Study the drawing (mm; zero at the part's minimum x, y, z) and answer. A direction names the side the tool comes from. Coordinates: 2 decimals unless noted, no trailing zeros. Write each loop counter-clockwise with the first axis right and the second up, starting at its lowest first coordinate (ties: lowest second). Pieces come first, ordered by that corner, then holes. Notation, with made-up numbers: M 84.25,59 L 101.25,59 A23 cw 101.25,98 Z; hole C 72.25,21.25 d6. An arc over 180 degrees is marked long. Answer as a JSON object with one key per item and string values. Group by question number.
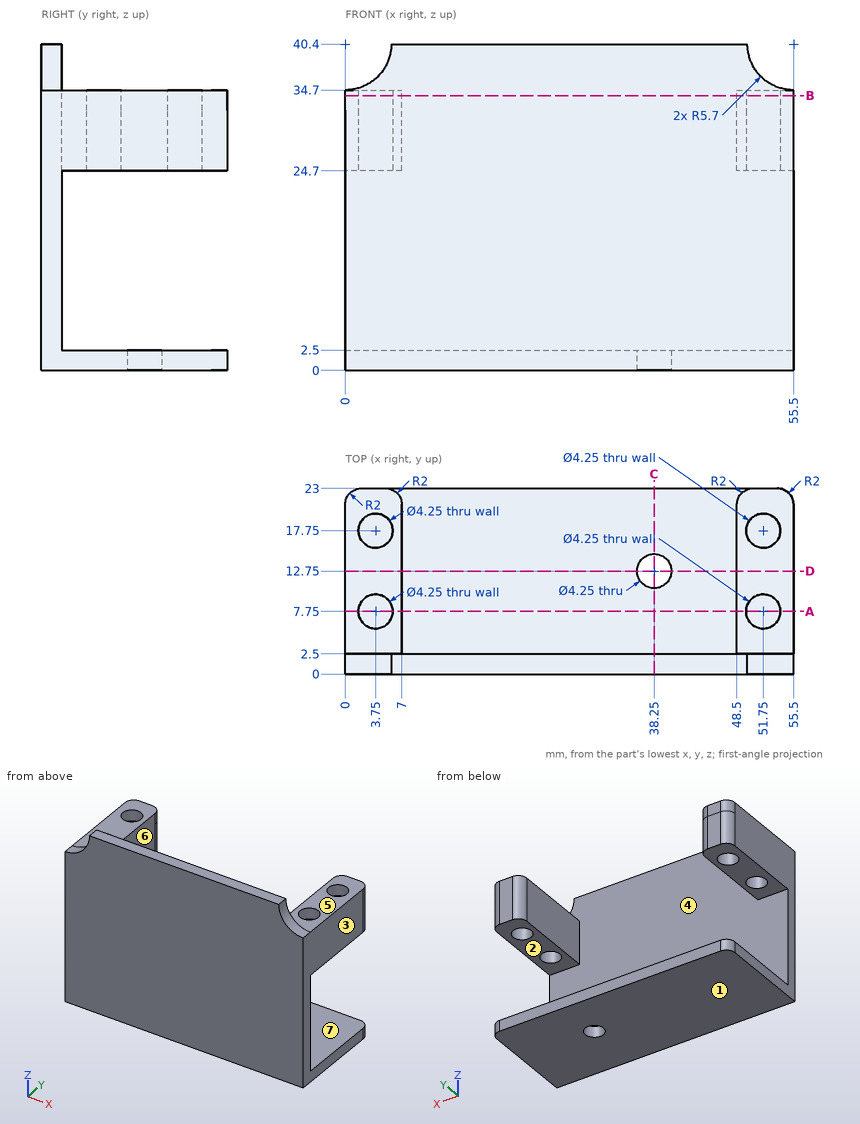
Item 1: Consider L1, parallel to X at y = 7.75, z = 26.5 (3 decimals); L2, parallel to Y at x = 3.75, z = 26.5 (3 decimals); L3, parallel to Z at x = 2, y = 4.25. Determine where each line is inside the solid, lowest interval first. Write a range as from..to.
Item 2: Flat-ended cylindrical pins translate along their axes: pin 1 Ø5.5 at (x, y) = (53, 9.5) entering from +Z; pin 2 Ø1 at (x, y) = (25, 4.5) entering from +Z; pin 3 Ø12 at (x, z) = (20.5, 15.5) entering from +Y. Find the tip coordinate at first contact, or state that the pin passes through.
Item 3: A cutting plane is placed at D-D, the plane y = 12.75. Write down the section's boundary in (x, z) (3 decimals), and give its area (3 significant figures).
Item 4: A cutting plane is placed at C-C, the plane x = 38.25. Write down the section's boundary in (y, z) (3 decimals).
Item 5: A tool of negligible diameter and unlimited length cuts with its end or side. For the marked faces 5, 6 and 7, from which of +Z, -Z, +X, -X, +Y, -Y can it reach the whole face along a straight path? Write none if from no direction.
Item 6: A cutting plane is placed at B-B, the plane z = 34. Write down the section's boundary in (x, y) (3 decimals), and give its area (3 significant figures).
Item 7: For a pull along Z with two mould halves and no side action, classify the marked faces 1, 2, 3 and 4 as +Z half, -Z half, draft (parallel to the pull), parting line (faces both ways), or undercut.
Item 8: A cutting plane is placed at A-A, the plane y = 7.75. Write down the section's boundary in (x, z) (3 decimals), and give its area (3 significant figures).
Answer:
{
 "1": {"L1": "0..1.625, 5.875..7, 48.5..49.625, 53.875..55.5", "L2": "0..5.625, 9.875..15.625, 19.875..23", "L3": "0..2.5, 24.7..34.7"},
 "2": {"pin 1": "z = 34.7", "pin 2": "z = 2.5", "pin 3": "y = 2.5"},
 "3": {"outline": "M 0,0 L 36.125,0 L 36.125,2.5 L 0,2.5 Z; M 0,24.7 L 7,24.7 L 7,34.7 L 0,34.7 Z; M 40.375,0 L 55.5,0 L 55.5,2.5 L 40.375,2.5 Z; M 48.5,24.7 L 55.5,24.7 L 55.5,34.7 L 48.5,34.7 Z", "area": "268 mm2"},
 "4": {"outline": "M 0,0 L 10.625,0 L 10.625,2.5 L 2.5,2.5 L 2.5,40.4 L 0,40.4 Z; M 14.875,0 L 23,0 L 23,2.5 L 14.875,2.5 Z"},
 "5": {"face 5": "+Z, +X, -X, +Y", "face 6": "+Z, +Y", "face 7": "+X, -X, +Y"},
 "6": {"outline": "M 0,0 L 55.5,0 L 55.5,21 A2 ccw 53.5,23 L 50.5,23 A2 ccw 48.5,21 L 48.5,2.5 L 7,2.5 L 7,21 A2 ccw 5,23 L 2,23 A2 ccw 0,21 Z; hole C 3.75,7.75 d4.25; hole C 3.75,17.75 d4.25; hole C 51.75,7.75 d4.25; hole C 51.75,17.75 d4.25", "area": "366 mm2"},
 "7": {"face 1": "-Z half", "face 2": "undercut", "face 3": "draft", "face 4": "undercut"},
 "8": {"outline": "M 0,0 L 55.5,0 L 55.5,2.5 L 0,2.5 Z; M 0,24.7 L 1.625,24.7 L 1.625,34.7 L 0,34.7 Z; M 5.875,24.7 L 7,24.7 L 7,34.7 L 5.875,34.7 Z; M 48.5,24.7 L 49.625,24.7 L 49.625,34.7 L 48.5,34.7 Z; M 53.875,24.7 L 55.5,24.7 L 55.5,34.7 L 53.875,34.7 Z", "area": "194 mm2"}
}
